Could you check a few things on this model? Use its own coordinates, in mm. A direction names the side the tool comes from. Coordinates: 2 decimals unless noted, no trailing zeros. Write each loop counter-clockwise with the first axis right and the second up, starting at its lowest first coordinate (ties: lowest second). Pieces come first, ordered by that corner, then holes. Notation, with made-up numbers: (-12, -6) - (39, -6) arc R8 ccw to (39, 5) - close; hole circle Ø6 at (77.25, 47). An arc over 180 degrees is marked (long way). Write item = value, one per line. Start each with the question number.
```python
from build123d import *

# Parameters (mm, degrees)
ESQUISSE1_W             = 50
ESQUISSE1_H             = 50
BOSS_EXTRU_1_DEPTH      = 50
ESQUISSE2_R             = 6
ENL_V_MAT_EXTRU_1_DEPTH = 40
CONG_1_R                = 10
ESQUISSE3_R             = 1.5
ENL_V_MAT_EXTRU_2_DEPTH = 21
ENL_V_MAT_EXTRU_3_DEPTH = 4
ESQUISSE5_R             = 1.75
ENL_V_MAT_EXTRU_4_DEPTH = 90


with BuildPart() as part:
    # Esquisse1 → Boss.-Extru.1 (new body)
    with BuildSketch(Plane.XY):
        with Locations((25, 25)):
            Rectangle(ESQUISSE1_W, ESQUISSE1_H)
    extrude(amount=BOSS_EXTRU_1_DEPTH)

    # Esquisse2 → Enlèv. mat.-Extru.1 (cut)
    with BuildSketch(Plane.ZY):
        with Locations((24.976890997, 24.856256207)):
            Circle(ESQUISSE2_R)
    extrude(amount=-ENL_V_MAT_EXTRU_1_DEPTH, mode=Mode.SUBTRACT)

    # Congé1
    cong_1_edges = [part.edges().sort_by_distance(p)[0] for p in [
        (25, 50, 50),
        (25, 50, 0),
        (25, 0, 0),
        (25, 0, 50),
    ]]
    fillet(cong_1_edges, radius=CONG_1_R)

    # Esquisse3 → Enlèv. mat.-Extru.2 (cut)
    with BuildSketch(Plane(origin=(0, 50, 0), x_dir=(1, 0, 0), z_dir=(0, 1, 0))):
        with Locations(Location((8.958242403, -24.894645172, 0), (0, 0, 270))):
            Circle(ESQUISSE3_R)
        with Locations(Location((27.695396355, -24.894645172, 0), (0, 0, 270))):
            Circle(ESQUISSE3_R)
    extrude(amount=-ENL_V_MAT_EXTRU_2_DEPTH, mode=Mode.SUBTRACT)

    # Esquisse4 → Enlèv. mat.-Extru.3 (cut)
    with BuildSketch(Plane(origin=(50, 0, 0), x_dir=(0, 0, -1), z_dir=(1, 0, 0))):
        with BuildLine():
            Line((-7.144655121, 28.135805281), (-18.224176514, 30.192846764))
            ThreePointArc((-18.224176514, 30.192846764), (-19.380476075, 30.704407729), (-20.091653936, 31.749849906))
            Line((-20.091653936, 31.749849906), (-22.148695418, 42.829371299))
            ThreePointArc((-22.148695418, 42.829371299), (-24.9999654, 45.1999956), (-27.851235382, 42.829371299))
            Line((-27.851235382, 42.829371299), (-29.908276864, 31.749849906))
            ThreePointArc((-29.908276864, 31.749849906), (-30.543285097, 30.543354297), (-31.749780706, 29.908346064))
            Line((-31.749780706, 29.908346064), (-42.829302099, 27.851304582))
            ThreePointArc((-42.829302099, 27.851304582), (-45.1999264, 25.0000346), (-42.829302099, 22.148764618))
            Line((-42.829302099, 22.148764618), (-31.749780706, 20.091723136))
            ThreePointArc((-31.749780706, 20.091723136), (-30.543285097, 19.456714903), (-29.908276864, 18.250219294))
            Line((-29.908276864, 18.250219294), (-27.851235382, 7.170697901))
            ThreePointArc((-27.851235382, 7.170697901), (-24.9999654, 4.8000736), (-22.148695418, 7.170697901))
            Line((-22.148695418, 7.170697901), (-20.091653936, 18.250219294))
            ThreePointArc((-20.091653936, 18.250219294), (-19.456645703, 19.456714903), (-18.250150094, 20.091723136))
            Line((-18.250150094, 20.091723136), (-7.170628701, 22.148764618))
            ThreePointArc((-7.170628701, 22.148764618), (-4.657744871, 25.131439646), (-7.144655121, 28.135805281))
        make_face()
    extrude(amount=-ENL_V_MAT_EXTRU_3_DEPTH, mode=Mode.SUBTRACT)

    # Esquisse5 → Enlèv. mat.-Extru.4 (cut)
    with BuildSketch(Plane(origin=(46, 0, 0), x_dir=(0, 0, -1), z_dir=(1, 0, 0))):
        with Locations(Location((-24.9999654, 25.0000346, 0), (0, 0, 90))):
            Circle(ESQUISSE5_R)
    extrude(amount=-ENL_V_MAT_EXTRU_4_DEPTH, mode=Mode.SUBTRACT)


solid = part.part
```
1) For P1, Ø7, axis at y = 24.86, z = 24.98, coming from the -X side; P2, Ø3, axis at y = 25, z = 25, coming from the -X side; P3, Ø2.5, axis at x = 27.7, z = 24.89, coming from the +Y side, each with a flat end and sliding along its axis, tell me the tip position at first contact or that it passes through.
2) Suppose I cut it at A-A on y = 41.5. Please give me the cut outline in (x, z).
3) If I drill on probe 1 along Z at (x, y) = (14, 22.5); probe 2 along Z at (x, y) = (46.5, 33); probe 3 along Y at (x, z) = (20, 26), over which ranges is the centre line in solid material (lowest first)? Write a range as [from, to].
4) Thinking about a two-plate mould opening in Y: for faces 4 (the cylindrical face through (25.35, 2.85, 46.99)), 5 (the flat face through (25, 50, 25)), 6 (the flat face through (48.028, 21.106, 12.788)), 7 (the cylindrical face through (8.38, 40.45, 26.28)), which applies, +Y half, -Y half, draft (parallel to the pull), parting line (faces both ways), or undercut?
5) Suppose I cut it at D-D on x = 41.5. Please give me the cut outline in (y, z).
6) Suppose I cut it at B-B on x = 36. Please give me the cut outline in (y, z), plus the area to 3 significant figures.
7) Which directions (+Z, -Z, +X, -X, +Y, -Y) give clear straight access to the entire face, cutting with the end or side of a thin tool? Please do faces 1 (the cylindrical face through (27.12, 40.45, 26.28)), 2 (the cylindrical face through (48.028, 19.443, 19.47)), 3 (the flat face through (25, 25, 0)).
8) Suppose I cut it at C-C on z = 5.5. Please give me the cut outline in (x, y), plus the area to 3 significant figures.
Reply:
q1.P1 = 40
q1.P2 = through
q1.P3 = 19.01
q2.outline = (0, 0.11) - (50, 0.11) - (50, 21.9) - (46, 21.9) - (46, 28.1) - (50, 28.1) - (50, 49.89) - (0, 49.89) - close; hole circle Ø3 at (8.96, 24.89); hole circle Ø3 at (27.7, 24.89)
q3.probe_1 = [0, 19.46], [30.49, 50]
q3.probe_2 = [0, 20.32], [29.68, 50]
q3.probe_3 = [0, 18.94], [30.77, 50]
q4.face_4 = -Y half
q4.face_5 = +Y half
q4.face_6 = undercut
q4.face_7 = draft
q5.outline = (0, 10) arc R10 ccw to (10, 0) - (40, 0) arc R10 ccw to (50, 10) - (50, 40) arc R10 ccw to (40, 50) - (10, 50) arc R10 ccw to (0, 40) - close; hole circle Ø3.5 at (25, 25)
q6.outline = (0, 10) arc R10 ccw to (10, 0) - (40, 0) arc R10 ccw to (50, 10) - (50, 40) arc R10 ccw to (40, 50) - (10, 50) arc R10 ccw to (0, 40) - close; hole circle Ø12 at (24.86, 24.98)
q6.area = 2,300 mm^2
q7.face_1 = +Y
q7.face_2 = +X
q7.face_3 = -Z, +X, -X, +Y, -Y
q8.outline = (0, 1.07) - (50, 1.07) - (50, 23.04) - (46, 23.04) - (46, 27.25) - (50, 27.25) - (50, 48.93) - (0, 48.93) - close
q8.area = 2,380 mm^2
